Autodesk Fusion 360 part; units mm, degrees
sketch "Sketch1" plane through (0, 0, 0) normal (0, 0, 1) x (1, 0, 0)
  circle A0 centre (0, 0) radius 40
  line L0 (0, 40) -> (0, -40) construction
  circle A1 centre (0, 0) radius 43
  line L1 (-26, 14.5) -> (-26, -14.5)
  line L2 (-40.4815, -14.5) -> (-26, -14.5)
  line L3 (-26, 14.5) -> (-40.4815, 14.5)
  line L4 (40, 0) -> (-40, 0) construction
  line L5 (26, 14.5) -> (40.4815, 14.5)
  line L6 (26, 14.5) -> (26, -14.5)
  line L7 (40.4815, -14.5) -> (26, -14.5)
  circle A2 centre (15, -9) radius 1.1
  circle A3 centre (15, 9) radius 1.1
  circle A4 centre (-15, -9) radius 1.1
  circle A5 centre (-15, 9) radius 1.1
  line L8 (-26, 14.5) -> (26, 14.5)
  line L9 (26, -14.5) -> (-26, -14.5)
  line L10 (17.5, -35.9687) -> (-17.5, -35.9687)
  dimension "d1" = 80
  dimension "d39" = 3
  dimension "d40" = 29
  dimension "d41" = 14
  dimension "d49" = 2.2
  dimension "d50" = 9
  dimension "d51" = 15
  dimension "d52" = 11
  dimension "d69" = 35
extrude "Extrude1" add sketch "Sketch1" along normal blind 4 contours A0 L10 | A0 L2 L7 L9 L10 | A0 L3 L5 L8 | L1 L6 L8 L9
sketch "Sketch3" plane through (0, 0, 4) normal (0, 0, 1) x (-1, 0, 0)
  circle A0 centre (0, 0) radius 38
  circle A1 centre (0, 0) radius 40
  line L0 (37.2794, -14.5) -> (26, -14.5)
  line L1 (26, -14.5) -> (26, 14.5)
  line L2 (26, 14.5) -> (37.2794, 14.5)
  line L3 (-26, 14.5) -> (-26, -14.5)
  line L4 (-26, -14.5) -> (-37.2794, -14.5)
  line L5 (-37.2794, 14.5) -> (-26, 14.5)
  circle A2 centre (-15, 9) radius 1.1
  circle A3 centre (15, -9) radius 1.1
  circle A4 centre (-15, -9) radius 1.1
  circle A5 centre (15, 9) radius 1.1
  arc A6 (-37.2794, -14.5) -> (37.2794, -14.5) centre (0, 0) ccw
  arc A7 (37.2794, 14.5) -> (-37.2794, 14.5) centre (0, 0) ccw
  dimension "d20" = 76
  dimension "d21" = 80
extrude "Extrude7" add sketch "Sketch3" along normal blind 80 and the other way blind 4 contours A0 A1 L0 L2 | A0 A1 L2 L5 A7 | A0 A1 L0 L4 A6 | A0 A1 L4 L5
extrude "Extrude12" add sketch "Sketch1" along normal blind 9 contours L1 L6 L8 L9
sketch "Sketch7" plane through (0, 0, 0) normal (0, 1, 0) x (1, 0, 0)
  line L0 (-15, -55) -> (15, -55)
  line L1 (15, -55) -> (15, -40)
  line L2 (15, -40) -> (-15, -40)
  line L3 (-15, -40) -> (-15, -55)
  line L4 (0, 0) -> (0, -80) construction
  line L5 (15, -40) -> (-15, -40)
  line L6 (-15, -40) -> (-15, -37)
  line L7 (-15, -37) -> (15, -37)
  line L8 (15, -37) -> (15, -40)
  dimension "d63" = 30
  dimension "d64" = 15
  dimension "d65" = 80
  dimension "d68" = 3
extrude "Extrude14" cut sketch "Sketch7" against normal blind 60 contours L0 L1 L2 L3 L5
extrude "Extrude15" add sketch "Sketch1" along normal blind 40 contours A0 L10
sketch "Sketch8" plane through (0, 0, 0) normal (1, 0, 0) x (0, 1, 0)
  circle A0 centre (0, 69) radius 4
  line L0 (40, 84) -> (-40, 84)
  dimension "d72" = 8
  dimension "d73" = 15
extrude "Extrude16" cut sketch "Sketch8" along normal blind 100
Verification items for the finished model (mm, model axes). A direction names the side the tool comes from. Give positions to 0.01 mm unless a question says otherwise; leave off trailing zeros. Order: outer loops, then holes, each group sorted by start corner. A loop starts at its lowest first (then second) coordinate and runs counter-clockwise, first axis right, second up. Notation, with made-up numbers: M 50.5,-21.5 L 104.5,-21.5 A6 cw 104.5,-14.5 Z; hole C 31.25,10 d10. An arc over 180 degrees is marked long. Answer as a JSON object with one key per item and string values. Group by question number.
1) Mould release check, pull along X, two halves, no side actions. Record for faces 1 (the face through (31, -14.5, 2)), 2 (the face through (-1, 1, 0)): released by +X, released by -X, zero draft, split by the parting line, or undercut.
2) Cross-section at C-C (z = 29.5). Enter the section's corners in (x, y), then the cut area to 3 significant figures.
3) Access from +Z, -Z, +X, -X, +Y, -Y to the whole of each face (thin tool, end or side, straight path). Record for faces 3 (the face through (-26, 0, 4)), 4 (the face through (0, -39, 55)), 5 (the face through (0, 24, 4)), 6 (the face through (39, -4, 69)).
4) Cross-section at A-A (x = 0). Enter the section's corners in (y, z).
5) Cross-section at D-D (x = 9.5). Enter the section's corners in (y, z).
6) Scan lines: line 1 along Y through (x, z) = (-15, 4.25); line 2 along X through (y, z) = (-1, 27); line 3 along Y through (x, z) = (-13.5, 7.5). Record each from-to range of solid material in increasing order. Write a range as [from, to].
7) Cross-section at B-B (y = 11.5). Enter the section's corners in (x, z).
8) Depth check by flat-ended pin: pin 1 Ø4 at (x, z) = (7.5, 6.5) entering from -Y; pin 2 Ø1.2 at (x, z) = (-32.5, 2.5) entering from -Y; pin 3 Ø6 at (x, z) = (-23.5, 30) entering from +Y; pin 4 Ø4 at (x, y) = (-5.5, -36) entering from -Z. Enter the tip coordinate at first touch or a pass-through.
Result sheet:
{
 "1": {"face 1": "undercut", "face 2": "zero draft"},
 "2": {"outline": "C 0,0 d80; hole M -12.26,-35.97 L 12.26,-35.97 A38 ccw long Z", "area": "523 mm2"},
 "3": {"face 3": "+Z, -Z", "face 4": "-Y", "face 5": "+Z", "face 6": "+X"},
 "4": {"outline": "M -40,0 L 40,0 L 40,84 L 38,84 L 38,4 L 14.5,4 L 14.5,9 L -14.5,9 L -14.5,4 L -35.97,4 L -35.97,40 L -40,40 Z; M -40,55 L -38,55 L -38,84 L -40,84 Z"},
 "5": {"outline": "M -38.86,0 L 38.86,0 L 38.86,84 L 36.79,84 L 36.79,4 L 14.5,4 L 14.5,9 L -14.5,9 L -14.5,4 L -35.97,4 L -35.97,40 L -38.86,40 Z; M -38.86,55 L -36.79,55 L -36.79,84 L -38.86,84 Z"},
 "6": {"line 1": "y = [-37.08, -34.91], [-14.5, -10.1], [-7.9, 7.9], [10.1, 14.5], [34.91, 37.08]", "line 2": "x = [-39.99, -37.99], [37.99, 39.99]", "line 3": "y = [-37.65, -35.52], [-14.5, 14.5], [35.52, 37.65]"},
 "7": {"outline": "M -38.31,0 L -36.22,0 L -36.22,84 L -38.31,84 Z; M -26,0 L 26,0 L 26,9 L -26,9 Z; M 36.22,0 L 38.31,0 L 38.31,84 L 36.22,84 Z"},
 "8": {"pin 1": "stops at y = -39.62", "pin 2": "stops at y = -24.13", "pin 3": "stops at y = 34.35", "pin 4": "stops at z = 0"}
}
